Check sheet for the modelled part. Datum: model origin and axes. Units: mm. Give positions to 0.01 mm unless a question says otherwise; leave off trailing zeros. Order: outer loops, then holes, each group sorted by start corner. A loop starts at its lowest first (then second) coordinate and runs counter-clockwise, first axis right, second up. Notation, with made-up numbers: (71, 3) -> (84, 3) arc R28 ccw to (84, 26) -> close; hole circle Ø10 at (22.25, 43). An arc over 180 degrees is marked (long way). Answer in a Markdown table with one row per item. Add a question column.
(1) Release check for a two-part mould opening along X. For faces 1 (the face through (20, -15, 0)), 2 (the face through (33.62, -14.49, 0.99)), 3 (the face through (0, -15, 1)) record: released by +X, released by -X, zero draft, split by the parting line, or undercut.
(2) Cross-section at D-D (y = -8.5). Record the cut outline in (x, z), then the cut area to 3 significant figures.
(3) Cross-section at A-A (z = 0.9). Record the cut outline in (x, y).
(4) Thickness scan on L1, parallel to X at y = -15, z = 1.2; L2, parallel to X at y = -15.5, z = 0.9; L3, parallel to Y at x = 32, z = 1.6. Record the ranges inside material, lowest first. Write a range as [from, to].
(5) Cross-section at B-B (x = 32). Record the cut outline in (y, z).
(6) Cross-section at C-C (y = -14.25). Record the cut outline in (x, z), then the cut area to 3 significant figures.
```python
from build123d import *

# Parameters (mm, degrees)
CYLINDER001_R     = 1.7
CYLINDER001_DEPTH = 10
CYLINDER_R        = 1.7
CYLINDER_DEPTH    = 10
BOX003_W          = 40
BOX003_H          = 15
BOX003_DEPTH      = 2
FILLET003_R       = 5


with BuildPart() as cylinder001:
    # Cylinder001 → Cylinder001 (new body)
    with BuildSketch(Plane(origin=(32, 0, 0), x_dir=(1, 0, 0), z_dir=(0, 0, 1))):
        Circle(CYLINDER001_R)
    extrude(amount=CYLINDER001_DEPTH)


with BuildPart() as cylinder:
    # Cylinder → Cylinder (new body)
    with BuildSketch(Plane(origin=(8, 0, 0), x_dir=(1, 0, 0), z_dir=(0, 0, 1))):
        Circle(CYLINDER_R)
    extrude(amount=CYLINDER_DEPTH)


with BuildPart() as union:
    # Box003 → Box003 (new body)
    with BuildSketch(Plane.XY):
        with Locations((20, 7.5)):
            Rectangle(BOX003_W, BOX003_H)
    extrude(amount=BOX003_DEPTH)

    # Fillet003
    fillet003_edges = [union.edges().sort_by_distance(p)[0] for p in [
        (0, 0, 1),
        (0, 15, 1),
        (40, 0, 1),
        (40, 15, 1),
    ]]
    fillet(fillet003_edges, radius=FILLET003_R)


with BuildPart() as union_1:
    # Fillet003 placement: moved
    add(union.part.moved(Location((0, -7.5, 0))))

    # Cut002: cut Cylinder
    add(cylinder.part, mode=Mode.SUBTRACT)

    # Cut003: cut Cylinder001
    add(cylinder001.part, mode=Mode.SUBTRACT)


with BuildPart() as union_2:
    # Cut003 placement: moved
    add(union_1.part.moved(Location((0, -15, 0))))


solid = union_2.part
```
Answer below:
| question | item | result |
|---|---|---|
| 1 | face 1 | zero draft |
| 1 | face 2 | undercut |
| 1 | face 3 | released by -X |
| 2 | outline | (2, 0) -> (38, 0) -> (38, 2) -> (2, 2) -> close |
| 2 | area | 72.0 mm² |
| 3 | outline | (0, -17.5) arc R5 ccw to (5, -22.5) -> (35, -22.5) arc R5 ccw to (40, -17.5) -> (40, -12.5) arc R5 ccw to (35, -7.5) -> (5, -7.5) arc R5 ccw to (0, -12.5) -> close; hole circle Ø3.4 at (8, -15); hole circle Ø3.4 at (32, -15) |
| 4 | L1 | x = [0, 6.3], [9.7, 30.3], [33.7, 40] |
| 4 | L2 | x = [0, 6.38], [9.62, 30.38], [33.62, 40] |
| 4 | L3 | y = [-22.5, -16.7], [-13.3, -7.5] |
| 5 | outline | (-22.5, 0) -> (-16.7, 0) -> (-16.7, 2) -> (-22.5, 2) -> close; (-13.3, 0) -> (-7.5, 0) -> (-7.5, 2) -> (-13.3, 2) -> close |
| 6 | outline | (0, 0) -> (6.47, 0) -> (6.47, 2) -> (0, 2) -> close; (9.53, 0) -> (30.47, 0) -> (30.47, 2) -> (9.53, 2) -> close; (33.53, 0) -> (40, 0) -> (40, 2) -> (33.53, 2) -> close |
| 6 | area | 67.8 mm² |
